Can you work these out from the model? Positions are in its coordinate system, mm. Give positions to 0.01 mm unless a question says otherwise; leave off trailing zeros. Order: outer loops, then holes, each group sorted by start corner. A loop starts at its lowest first (then second) coordinate and runs counter-clockwise, first axis right, second up. Notation, with made-up numbers: (83, -12.75) -> (92, -12.75) arc R18 cw to (92, 13.25) -> close; hole circle Ø2 at (73, 7.5). An arc over 180 degrees is marked (long way). Answer as a JSON object with one key per item and string values.
Autodesk Inventor part; units mm, degrees
ref_plane "YZ Plane" through (0, 0, 0) normal (1, 0, 0) x (0, 1, 0)
ref_plane "XZ Plane" through (0, 0, 0) normal (0, 1, 0) x (-1, 0, 0)
ref_plane "XY Plane" through (0, 0, 0) normal (0, 0, 1) x (1, 0, 0)
sketch "Sketch1" plane through (0, 0, 0) normal (0, 1, 0) x (-1, 0, 0)
  line L0 (0, 0) -> (-76.2, 0)
  line L1 (-76.2, 0) -> (-76.2, -76.2)
  line L2 (-76.2, -76.2) -> (0, -76.2)
  line L3 (0, -76.2) -> (0, 0)
  line L4 (-44.45, -73.66) -> (-31.75, -73.66)
  line L5 (-31.75, -73.66) -> (-31.75, -68.834)
  line L6 (-31.75, -68.834) -> (-44.45, -68.834)
  line L7 (-44.45, -68.834) -> (-44.45, -73.66)
  line L8 (-68.834, -31.75) -> (-68.834, -44.45)
  line L9 (-68.834, -44.45) -> (-73.66, -44.45)
  line L10 (-73.66, -31.75) -> (-68.834, -31.75)
  line L11 (-73.66, -44.45) -> (-73.66, -31.75)
  line L12 (-7.366, -44.45) -> (-2.54, -44.45)
  line L13 (-7.366, -31.75) -> (-7.366, -44.45)
  line L14 (-2.54, -44.45) -> (-2.54, -31.75)
  line L15 (-2.54, -31.75) -> (-7.366, -31.75)
  line L16 (-44.45, -2.54) -> (-31.75, -2.54)
  line L17 (-31.75, -2.54) -> (-31.75, -7.366)
  line L18 (-31.75, -7.366) -> (-44.45, -7.366)
  line L19 (-44.45, -7.366) -> (-44.45, -2.54)
  circle A0 centre (-38.1, -38.1) radius 11.43
  dimension "d0" = 76.2
  dimension "d1" = 76.2
  dimension "d6" = 31.75
  dimension "d7" = 2.54
  dimension "d8" = 4.826
  dimension "d9" = 12.7
  dimension "d15" = 31.75
  dimension "d16" = 12.7
  dimension "d17" = 4.826
  dimension "d18" = 22.86
extrude "Extrusion3" add sketch "Sketch1" along normal blind 4.826
fillet "Fillet1" radius 3.175 4 edges at (76.2, 2.413, 0) (0, 2.413, 0) (76.2, 2.413, -76.2) (0, 2.413, -76.2)
properties part number "top"
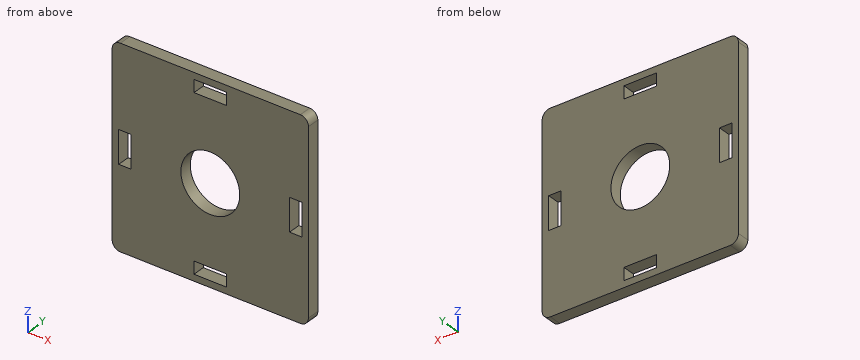
1. If we section it at B-B on y = 2: Please give me the cut outline in (x, z) (3 decimals).
Worked answers:
{"outline": "(0, -73.025) arc R3.175 ccw to (3.175, -76.2) -> (73.025, -76.2) arc R3.175 ccw to (76.2, -73.025) -> (76.2, -3.175) arc R3.175 ccw to (73.025, 0) -> (3.175, 0) arc R3.175 ccw to (0, -3.175) -> close; hole (2.54, -44.45) -> (7.366, -44.45) -> (7.366, -31.75) -> (2.54, -31.75) -> close; hole circle Ø22.86 at (38.1, -38.1); hole (31.75, -73.66) -> (44.45, -73.66) -> (44.45, -68.834) -> (31.75, -68.834) -> close; hole (31.75, -7.366) -> (44.45, -7.366) -> (44.45, -2.54) -> (31.75, -2.54) -> close; hole (68.834, -44.45) -> (73.66, -44.45) -> (73.66, -31.75) -> (68.834, -31.75) -> close"}
2. If we section it at D-D on x = 72: Please give me the cut outline in (y, z), then the cut area to 3 significant figures.
Worked answers:
{"outline": "(0, -76.2) -> (4.83, -76.2) -> (4.83, -44.45) -> (0, -44.45) -> close; (0, -31.75) -> (4.83, -31.75) -> (4.83, 0) -> (0, 0) -> close", "area": "306 mm²"}
3. If we section it at A-A on x = 38.1: Please give me the cut outline in (y, z).
Worked answers:
{"outline": "(0, -76.2) -> (4.83, -76.2) -> (4.83, -73.66) -> (0, -73.66) -> close; (0, -68.83) -> (4.83, -68.83) -> (4.83, -49.53) -> (0, -49.53) -> close; (0, -26.67) -> (4.83, -26.67) -> (4.83, -7.37) -> (0, -7.37) -> close; (0, -2.54) -> (4.83, -2.54) -> (4.83, 0) -> (0, 0) -> close"}
4. If we section it at C-C on z = -38.1: Please give me the cut outline in (x, y).
Worked answers:
{"outline": "(0, 0) -> (2.54, 0) -> (2.54, 4.83) -> (0, 4.83) -> close; (7.37, 0) -> (26.67, 0) -> (26.67, 4.83) -> (7.37, 4.83) -> close; (49.53, 0) -> (68.83, 0) -> (68.83, 4.83) -> (49.53, 4.83) -> close; (73.66, 0) -> (76.2, 0) -> (76.2, 4.83) -> (73.66, 4.83) -> close"}
5. Will this pin go through, and if not, where does the flat tip stop? pin 1 Ø1.4 at (x, y) = (41, 3.5) entering from +Z.
Worked answers:
{"pin 1": "z = 0"}
6. Please list where these lines run through material, in increasing order: L1, parallel to Z at x = 38.1, y = 3.35; L2, parallel to Z at x = 6, y = 4.25; L3, parallel to Z at x = 34.5, y = 2.3.
Worked answers:
{"L1": "-76.2 to -73.66, -68.83 to -49.53, -26.67 to -7.37, -2.54 to 0", "L2": "-76.2 to -44.45, -31.75 to 0", "L3": "-76.2 to -73.66, -68.83 to -48.95, -27.25 to -7.37, -2.54 to 0"}
